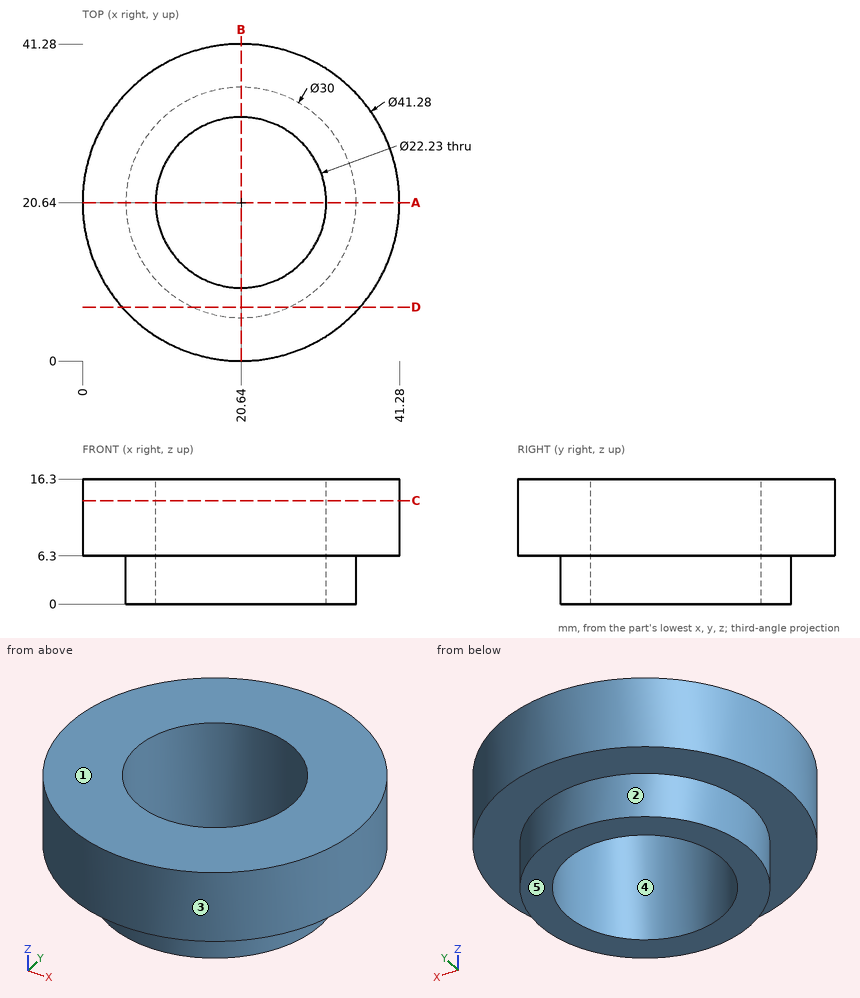
Check sheet for the drawn part. Datum: minimum x, y, z corner. Units: mm. A direction names the side the tool comes from. Give positions to 0.01 mm unless a question says otherwise; leave off trailing zeros. Write each loop counter-clockwise with the first axis right and the second up, starting at its lowest first coordinate (ties: lowest second). Pieces come first, ordered by that corner, then holes. Notation, with made-up numbers: (60, -1.75) - (89, -1.75) arc R20 ccw to (89, 8.25) - close; hole circle Ø11 at (45.5, 75.5). An arc over 180 degrees is marked (long way). Put each result on its own line as item: value.
1. Sectioned sample at A-A, the plane y = 20.64. Enter the section's corners in (x, z) (3 decimals), plus the area to 3 significant figures.
Ans:
outline: (0, 6.3) - (5.64, 6.3) - (5.64, 0) - (9.525, 0) - (9.525, 16.3) - (0, 16.3) - close; (31.755, 0) - (35.64, 0) - (35.64, 6.3) - (41.28, 6.3) - (41.28, 16.3) - (31.755, 16.3) - close
area: 239 mm²
2. Go/stop test with flat-tipped pins: pin 1 (1.5 mm diameter, centred on x = 31.5, y = 32.5, fed in from -Z); pin 2 (8 mm diameter, centred on x = 32.5, z = 9.5, fed in from +Y). Record where each tip stops, or that it passes through.
Ans:
pin 1: stops at z = 6.3
pin 2: stops at y = 39.72
3. Draft check along X on the marked faces 3, 4 and 5. Enter one of: +X half, -X half, draft (parallel to the pull), parting line (faces both ways), or undercut.
Ans:
face 3: parting line
face 4: undercut
face 5: draft
4. Set-up check for the marked faces 1 and 2: record each of +Z, -Z, +X, -X, +Y, -Y from which the full face is reachable in a straight line by a thin tool's end or side.
Ans:
face 1: +Z, +X, -X, +Y, -Y
face 2: -Z
5. Thickness scan on line 1 (Y direction, x = 20.64, z = 6) (3 decimals); line 2 (Y direction, x = 20.64, z = 6.5) (3 decimals); line 3 (Z direction, x = 36, y = 12.5). Record the ranges inside material, lowest first.
Ans:
line 1: y = 5.64 to 9.525, 31.755 to 35.64
line 2: y = 0 to 9.525, 31.755 to 41.28
line 3: z = 6.3 to 16.3
6. Sectioned sample at D-D, the plane y = 7. Enter the section's corners in (x, z).
Ans:
outline: (5.15, 6.3) - (14.4, 6.3) - (14.4, 0) - (26.88, 0) - (26.88, 6.3) - (36.13, 6.3) - (36.13, 16.3) - (5.15, 16.3) - close
7. Sectioned sample at C-C, the plane z = 13.5. Enter the section's corners in (x, y) (3 decimals), plus the area to 3 significant figures.
Ans:
outline: circle Ø41.28 at (20.64, 20.64); hole circle Ø22.23 at (20.64, 20.64)
area: 950 mm²
